Source: CAD feature listing. Evaluate the final solid. Frame: model axes, mm. A direction names the side the tool comes from. Give positions to 0.01 mm unless a question says otherwise; leave off trailing zeros. Loops run counter-clockwise (first coordinate to the right, second up) from the corner with the lowest first, then second, coordinate; pieces in that order, holes last. Notation, with made-up numbers: (-10.75, -15.5) -> (6.25, -15.5) arc R5 ccw to (6.25, -10.5) -> close; hole circle Ø7 at (-29.5, 18.25). An arc over 180 degrees is marked (long way). Return JSON: item names as keys, results as strings. Group by question number.
(1) Draft query along Y for faces 1 (the face through (2, 64, 19.05)), 2 (the face through (2, 38, 6.35)), 3 (the face through (144.67, 66.81, 0.27)). Return one class per face: released by +Y, released by -Y, zero draft, split by the parting line, or undercut.
(2) Pin query (flat end, axial travel): pin 1 (11.5 mm diameter, centred on x = -30, z = -2, fed in from +Y); pin 2 (19 mm diameter, centred on x = 38, y = 36, fed in from +Z); pin 3 (2 mm diameter, centred on y = 93.5, z = 2, fed in from -X). Return the tip coordinate at first contact, or that it passes through.
(3) Access query for faces 4 (the face through (5.796, 98.114, 7.559)), 5 (the face through (2, 39, -19.05)). Directions: +Z, -Z, +X, -X, +Y, -Y. A direction counts if a zero-diameter tool reaches every point of the face in a straight line with its end or side. Return the directions, or none.
(4) Ray query, line 1 (Z direction, x = -59, y = 40); line 2 (Y direction, x = -123.5, z = -2); line 3 (Y direction, x = -115, z = 13.5). Return the intervals inside material, ascending. Write a range as from..to.
(5) Cut plane A-A on z = 3.5. Return loops of the section in (x, y).
(6) Cut plane C-C on y = 62.5. Return loops of the section in (x, z), then the cut area to 3 significant figures.
(7) Cut plane D-D on y = 87. Return loops of the section in (x, z) (3 decimals).
(8) Cut plane B-B on y = 7. Return loops of the section in (x, z).
```python
from build123d import *

# Parameters (mm, degrees)
BOSS_EXTRUDE1_DEPTH = 19.05
CUT_EXTRUDE1_DEPTH  = 12.7
CUT_EXTRUDE1_TAPER  = 25
SKETCH9_R           = 9.525
BOSS_EXTRUDE3_DEPTH = 44.45


with BuildPart() as part:
    # Sketch2 → Boss-Extrude1 (new, symmetric)
    with BuildSketch(Plane.XY):
        Polygon((-137.16, 76.2), (137.16, 76.2), (152.4, 57.15), (152.4, 19.05), (137.16, 0), (-137.16, 0), (-152.4, 19.05), (-152.4, 57.15), align=None)
    extrude(amount=BOSS_EXTRUDE1_DEPTH, both=True)

    # 3DSketch1 → Cut-Extrude1 (cut)
    with BuildSketch(Plane(origin=(127.393703099, 20.32, 19.05), x_dir=(-0.9935119261035652, 0.11372797672509682, 0), z_dir=(0, 0, -1))):
        Polygon((0, 0), (253.134326679, -28.976456202), (258.45642237, -23.689554441), (261.16818156, 0), (257.178493531, 6.35282789), (4.044166852, 35.329284092), (-1.277928839, 30.042382332), (-3.989688029, 6.35282789), align=None)
    extrude(amount=CUT_EXTRUDE1_DEPTH, taper=CUT_EXTRUDE1_TAPER, mode=Mode.SUBTRACT)

    # Sketch9 → Boss-Extrude3 (add)
    with BuildSketch(Plane(origin=(0, 76.2, 0), x_dir=(1, 0, 0), z_dir=(0, 1, 0))):
        with Locations(Location((0, 0, 0), (0, 0, 90))):
            Circle(SKETCH9_R)
    extrude(amount=BOSS_EXTRUDE3_DEPTH)


solid = part.part
```
Answers:
{
 "1": {"face 1": "zero draft", "face 2": "undercut", "face 3": "released by +Y"},
 "2": {"pin 1": "y = 76.2", "pin 2": "z = 6.35", "pin 3": "x = -9.47"},
 "3": {"face 4": "+Y", "face 5": "-Z, +X, -X, +Y, -Y"},
 "4": {"line 1": "-19.05..6.35", "line 2": "0..76.2", "line 3": "0..22.91, 53.29..76.2"},
 "5": {"outline": "(-152.4, 19.05) -> (-137.16, 0) -> (137.16, 0) -> (152.4, 19.05) -> (152.4, 57.15) -> (137.16, 76.2) -> (8.86, 76.2) -> (8.86, 120.65) -> (-8.86, 120.65) -> (-8.86, 76.2) -> (-137.16, 76.2) -> (-152.4, 57.15) -> close"},
 "6": {"outline": "(-148.12, -19.05) -> (148.12, -19.05) -> (148.12, 19.05) -> (-148.12, 19.05) -> close", "area": "11,300 mm²"},
 "7": {"outline": "circle Ø19.05 at (0, 0)"},
 "8": {"outline": "(-142.76, -19.05) -> (142.76, -19.05) -> (142.76, 19.05) -> (-142.76, 19.05) -> close"}
}
